Geometry: final body of the model. Coordinates: model frame, mm. Give positions to 0.01 mm unless a question says otherwise; leave off trailing zeros. Order: outer loops, then holes, each group sorted by start corner. A loop starts at its lowest first (then second) coordinate and runs counter-clockwise, first axis right, second up. Notation, with made-up numbers: (66.5, -14) - (108.5, -14) arc R35 ccw to (108.5, 22) - close; hole circle Ø11 at (11, 29). An arc over 180 degrees is marked (long way). Write item = value, one per line. Start each with the question number.
Autodesk Inventor part; units mm, degrees
ref_plane "YZ Plane" through (0, 0, 0) normal (1, 0, 0) x (0, 1, 0)
ref_plane "XZ Plane" through (0, 0, 0) normal (0, 1, 0) x (-1, 0, 0)
ref_plane "XY Plane" through (0, 0, 0) normal (0, 0, 1) x (1, 0, 0)
sketch "Sketch1" plane through (0, 0, 0) normal (0, 0, 1) x (1, 0, 0)
  line L0 (21.5007, 49.9294) -> (-21.5007, 49.9294)
  line L1 (-21.5007, 49.9294) -> (-21.5007, -49.9294)
  line L2 (-21.5007, -49.9294) -> (21.5007, -49.9294)
  line L3 (21.5007, -49.9294) -> (21.5007, 49.9294)
  line L4 (-13.5007, 14.9765) -> (-16.5007, 14.9765)
  line L5 (-16.5007, 14.9765) -> (-16.5007, 27.3029)
  line L6 (-16.5007, 27.3029) -> (-13.5007, 27.3029)
  line L7 (-13.5007, 27.3029) -> (-13.5007, 14.9765)
  line L8 (-13.5007, -27.3029) -> (-16.5007, -27.3029)
  line L9 (-16.5007, -27.3029) -> (-16.5007, -14.9765)
  line L10 (-16.5007, -14.9765) -> (-13.5007, -14.9765)
  line L11 (-13.5007, -14.9765) -> (-13.5007, -27.3029)
  line L12 (-13.5007, -44.9294) -> (-16.5007, -44.9294)
  line L13 (-16.5007, -44.9294) -> (-16.5007, -32.6029)
  line L14 (-16.5007, -32.6029) -> (-13.5007, -32.6029)
  line L15 (-13.5007, -32.6029) -> (-13.5007, -44.9294)
  line L16 (-16.5007, 44.9294) -> (-13.5007, 44.9294)
  line L17 (-13.5007, 44.9294) -> (-13.5007, 32.6029)
  line L18 (-13.5007, 32.6029) -> (-16.5007, 32.6029)
  line L19 (-16.5007, 32.6029) -> (-16.5007, 44.9294)
  line L20 (-10.5007, -11.2324) -> (-13.5007, -11.2324)
  line L21 (-13.5007, -11.2324) -> (-13.5007, 11.2324)
  line L22 (-13.5007, 11.2324) -> (-10.5007, 11.2324)
  line L23 (-10.5007, 11.2324) -> (-10.5007, -11.2324)
  line L24 (16.5007, 14.9765) -> (13.5007, 14.9765)
  line L25 (13.5007, 14.9765) -> (13.5007, 27.3029)
  line L26 (13.5007, 27.3029) -> (16.5007, 27.3029)
  line L27 (16.5007, 27.3029) -> (16.5007, 14.9765)
  line L28 (16.5007, -27.3029) -> (13.5007, -27.3029)
  line L29 (13.5007, -27.3029) -> (13.5007, -14.9765)
  line L30 (13.5007, -14.9765) -> (16.5007, -14.9765)
  line L31 (16.5007, -14.9765) -> (16.5007, -27.3029)
  line L32 (16.5007, -44.9294) -> (13.5007, -44.9294)
  line L33 (13.5007, -44.9294) -> (13.5007, -32.6029)
  line L34 (13.5007, -32.6029) -> (16.5007, -32.6029)
  line L35 (16.5007, -32.6029) -> (16.5007, -44.9294)
  line L36 (13.5007, 44.9294) -> (16.5007, 44.9294)
  line L37 (16.5007, 44.9294) -> (16.5007, 32.6029)
  line L38 (16.5007, 32.6029) -> (13.5007, 32.6029)
  line L39 (13.5007, 32.6029) -> (13.5007, 44.9294)
  line L40 (4.1498, 36.9294) -> (4.1498, 39.9294)
  line L41 (4.1498, 39.9294) -> (9.5001, 39.9294)
  line L42 (9.5001, 39.9294) -> (9.5001, 36.9294)
  line L43 (9.5001, 36.9294) -> (4.1498, 36.9294)
  line L44 (-6.5006, 36.9294) -> (-6.5006, 39.9294)
  line L45 (-6.5006, 39.9294) -> (-1.1502, 39.9294)
  line L46 (-1.1502, 39.9294) -> (-1.1502, 36.9294)
  line L47 (-1.1502, 36.9294) -> (-6.5006, 36.9294)
  line L48 (-1.1502, 11.9294) -> (-1.1502, 8.9294)
  line L49 (-1.1502, 8.9294) -> (-6.5006, 8.9294)
  line L50 (-6.5006, 8.9294) -> (-6.5006, 11.9294)
  line L51 (-6.5006, 11.9294) -> (-1.1502, 11.9294)
  line L52 (9.5001, 11.9294) -> (9.5001, 8.9294)
  line L53 (9.5001, 8.9294) -> (4.1498, 8.9294)
  line L54 (4.1498, 8.9294) -> (4.1498, 11.9294)
  line L55 (4.1498, 11.9294) -> (9.5001, 11.9294)
  line L56 (4.1498, -11.9294) -> (4.1498, -8.9294)
  line L57 (4.1498, -8.9294) -> (9.5001, -8.9294)
  line L58 (9.5001, -8.9294) -> (9.5001, -11.9294)
  line L59 (9.5001, -11.9294) -> (4.1498, -11.9294)
  line L60 (-6.5006, -11.9294) -> (-6.5006, -8.9294)
  line L61 (-6.5006, -8.9294) -> (-1.1502, -8.9294)
  line L62 (-1.1502, -8.9294) -> (-1.1502, -11.9294)
  line L63 (-1.1502, -11.9294) -> (-6.5006, -11.9294)
  line L64 (4.1498, -39.9294) -> (4.1498, -36.9294)
  line L65 (4.1498, -36.9294) -> (9.5001, -36.9294)
  line L66 (9.5001, -36.9294) -> (9.5001, -39.9294)
  line L67 (9.5001, -39.9294) -> (4.1498, -39.9294)
  line L68 (-6.5006, -39.9294) -> (-6.5006, -36.9294)
  line L69 (-6.5006, -36.9294) -> (-1.1502, -36.9294)
  line L70 (-1.1502, -36.9294) -> (-1.1502, -39.9294)
  line L71 (-1.1502, -39.9294) -> (-6.5006, -39.9294)
  circle A0 centre (1.4998, 38.4294) radius 1.4
  line L72 (1.4998, 41.6656) -> (1.4998, 35.5125) construction
  circle A1 centre (1.4998, 10.4294) radius 1.4
  circle A2 centre (1.4998, -10.4294) radius 1.4
  circle A3 centre (1.4998, -38.4294) radius 1.4
  line L73 (-16.5007, 29.9529) -> (-13.5007, 29.9529) construction
  circle A4 centre (-15.0007, 29.9529) radius 1.4
  circle A5 centre (15.0007, 29.9529) radius 1.4
  line L74 (-16.5007, -29.9529) -> (-13.6007, -29.9529) construction
  circle A6 centre (-15.0507, -29.9529) radius 1.4
  circle A7 centre (15.0007, -29.9529) radius 1.4
  circle A8 centre (1.5007, -24.4294) radius 6.096
  circle A9 centre (1.5007, 24.4294) radius 6.096
  circle A10 centre (0, 0) radius 1.25
  dimension "d5" = 99.8588
  dimension "d6" = 43.0015
  dimension "d7" = 2.8
  dimension "d8" = 5.3
  dimension "d9" = 2.65
  dimension "d10" = 2.8
  dimension "d11" = 2.8
  dimension "d12" = 2.8
  dimension "d13" = 2.8
  dimension "d14" = 2.8
  dimension "d15" = 5.3
  dimension "d16" = 2.65
  dimension "d17" = 5.3
  dimension "d18" = 2.65
  dimension "d19" = 2.8
  dimension "d20" = 2.8
  dimension "d22" = 2.5
extrude "Extrusion1" add sketch "Sketch1" along normal blind 3
equation "\"d9\" = 0.5 * d8"
equation "\"d16\" = 0.5 * d15"
equation "\"d18\" = 0.5 * d17"
properties part number "X-Anchor-Side"
Q1. Section D-D, the plane z = 1.75. Count the separate pieces of the cut face and the enclosed holes in it, then the cut area to 3 significant figures.
Q2. Material intervals for line 1 along X through (y, z) = (-42, 0.9); line 2 along Y through (x, z) = (-5, 2.95); line 3 along X through (y, z) = (20.5, 2.1), sorted ascending. Write a range as from..to.
Q3. Pull-direction query (Y, two-part tool) for faces 1 (the cylindrical face through (14.7, 31.32, 1.48)), 2 (the flat face through (-5, 1, 0)); classes: +Y half, -Y half, draft (parallel to the pull), parting line (faces both ways), or undercut.
Q4. Section C-C, the plane y = 19.5. Return the cut outline in (x, z), then the cut area to 3 significant figures.
Q5. Section A-A, the plane y = 0. Return the cut outline in (x, z).
Q6. Section B-B, the plane x = 6. Return the cut outline in (y, z), then the cut area to 3 significant figures.
The answers:
q1.separate_pieces = 1
q1.enclosed_holes = 28
q1.area = 3,510 mm²
q2.line_1 = -21.5..-16.5, -13.5..13.5, 16.5..21.5
q2.line_2 = -49.93..-39.93, -36.93..-11.93, -8.93..8.93, 11.93..36.93, 39.93..49.93
q2.line_3 = -21.5..-16.5, -13.5..-3.16, 6.16..13.5, 16.5..21.5
q3.face_1 = undercut
q3.face_2 = draft
q4.outline = (-21.5, 0) - (-16.5, 0) - (-16.5, 3) - (-21.5, 3) - close; (-13.5, 0) - (-2.09, 0) - (-2.09, 3) - (-13.5, 3) - close; (5.09, 0) - (13.5, 0) - (13.5, 3) - (5.09, 3) - close; (16.5, 0) - (21.5, 0) - (21.5, 3) - (16.5, 3) - close
q4.area = 89.5 mm²
q5.outline = (-21.5, 0) - (-13.5, 0) - (-13.5, 3) - (-21.5, 3) - close; (-10.5, 0) - (-1.25, 0) - (-1.25, 3) - (-10.5, 3) - close; (1.25, 0) - (21.5, 0) - (21.5, 3) - (1.25, 3) - close
q6.outline = (-49.93, 0) - (-39.93, 0) - (-39.93, 3) - (-49.93, 3) - close; (-36.93, 0) - (-28.54, 0) - (-28.54, 3) - (-36.93, 3) - close; (-20.32, 0) - (-11.93, 0) - (-11.93, 3) - (-20.32, 3) - close; (-8.93, 0) - (8.93, 0) - (8.93, 3) - (-8.93, 3) - close; (11.93, 0) - (20.32, 0) - (20.32, 3) - (11.93, 3) - close; (28.54, 0) - (36.93, 0) - (36.93, 3) - (28.54, 3) - close; (39.93, 0) - (49.93, 0) - (49.93, 3) - (39.93, 3) - close
q6.area = 214 mm²
